from build123d import *

# Parameters (mm, degrees)
SKETCH1_W           = 38
SKETCH1_H           = 60
SKETCH1_R           = 1.5
SKETCH1_R_2         = 15.5
SKETCH1_R_3         = 1.2
BOSS_EXTRUDE1_DEPTH = 6.35


with BuildPart() as part:
    # Sketch1 → Boss-Extrude1 (new body)
    with BuildSketch(Plane(origin=(0, 0, 0), x_dir=(1, 0, 0), z_dir=(0, 1, 0))):
        with Locations((19, 30)):
            Rectangle(SKETCH1_W, SKETCH1_H)
        with Locations(Location((4, 4.05, 0), (0, 0, 270))):
            Circle(SKETCH1_R, mode=Mode.SUBTRACT)
        with Locations(Location((34, 4.05, 0), (0, 0, 270))):
            Circle(SKETCH1_R, mode=Mode.SUBTRACT)
        with Locations(Location((34, 34.05, 0), (0, 0, 270))):
            Circle(SKETCH1_R, mode=Mode.SUBTRACT)
        with Locations(Location((4, 34.05, 0), (0, 0, 270))):
            Circle(SKETCH1_R, mode=Mode.SUBTRACT)
        with Locations(Location((19, 19.05, 0), (0, 0, 270))):
            Circle(SKETCH1_R_2, mode=Mode.SUBTRACT)
        with Locations(Location((4, 56, 0), (0, 0, 270))):
            Circle(SKETCH1_R_3, mode=Mode.SUBTRACT)
        with Locations(Location((34, 56, 0), (0, 0, 270))):
            Circle(SKETCH1_R_3, mode=Mode.SUBTRACT)
    extrude(amount=BOSS_EXTRUDE1_DEPTH)


solid = part.part
CAD build for the part. Positions are in the model's coordinates, mm. Give positions to 0.01 mm unless a question says otherwise; leave off trailing zeros. Loops run counter-clockwise (first coordinate to the right, second up) from the corner with the lowest first, then second, coordinate; pieces in that order, holes last. Notation, with made-up numbers: M -4,24 L 10,24 A11 cw 10,35 Z; hole C -8,89.25 d8. An arc over 180 degrees is marked long. Write each question's results on one line, items separated by ' | '.
Q1. Mould opens along Z. For faces 1 (the face through (19, 3, 0)), 2 (the face through (33.09, 3.13, -35.24)), 3 (the face through (3.09, 3.13, -35.24)), 4 (the face through (38, 3, -30)) say: pulls with the +Z half, pulls with the -Z half, needs draft (parallel to the pull), parting line crosses it, or undercut.
Geometry check:
face 1: pulls with the +Z half | face 2: undercut | face 3: undercut | face 4: needs draft
Q2. Band-saw the part on B-B on x = 19. Write the cut outline in (y, z), and give its area (3 significant figures).
Geometry check:
outline: M 0,-60 L 6.35,-60 L 6.35,-34.55 L 0,-34.55 Z; M 0,-3.55 L 6.35,-3.55 L 6.35,0 L 0,0 Z | area: 184 mm²
Q3. Band-saw the part on D-D on z = -19.5. Write the cut outline in (x, y).
Geometry check:
outline: M 0,0 L 3.51,0 L 3.51,6.35 L 0,6.35 Z; M 34.49,0 L 38,0 L 38,6.35 L 34.49,6.35 Z
Q4. Band-saw the part on C-C on y = 4. Write the cut outline in (x, z), and give its area (3 significant figures).
Geometry check:
outline: M 0,-60 L 38,-60 L 38,0 L 0,0 Z; hole C 4,-34.05 d3; hole C 4,-4.05 d3; hole C 4,-56 d2.4; hole C 19,-19.05 d31; hole C 34,-34.05 d3; hole C 34,-4.05 d3; hole C 34,-56 d2.4 | area: 1,490 mm²
Q5. Probe probe 1 along X at (y, z) = (4.25, -56); probe 2 along X at (y, z) = (1.75, -5); probe 3 along Z at (x, y) = (5, 4.25). List the from-to ranges inside material, lowest first.
Geometry check:
probe 1: x = 0 to 2.8, 5.2 to 32.8, 35.2 to 38 | probe 2: x = 0 to 2.84, 5.16 to 12.45, 25.55 to 32.84, 35.16 to 38 | probe 3: z = -60 to -56.66, -55.34 to -35.17, -32.93 to -25.7, -12.4 to -5.17, -2.93 to 0
Q6. Flat gauge pin, fed straight in: P1, Ø2.5, axis at x = 34, z = -34.05, coming from the -Y side. Where does the tip first touch, or does it go through?
Geometry check:
P1: passes through
Q7. Band-saw the part on A-A on z = -56. Write the cut outline in (x, y), and give its area (3 significant figures).
Geometry check:
outline: M 0,0 L 2.8,0 L 2.8,6.35 L 0,6.35 Z; M 5.2,0 L 32.8,0 L 32.8,6.35 L 5.2,6.35 Z; M 35.2,0 L 38,0 L 38,6.35 L 35.2,6.35 Z | area: 211 mm²
